```python
from build123d import *

# Parameters (mm, degrees)
ESQUISSE1_R             = 20
ESQUISSE1_R_2           = 17
ESQUISSE1_R_3           = 15
BOSS_EXTRU_1_DEPTH      = 7.5
ESQUISSE1_3_R           = 15
ESQUISSE1_3_R_2         = 4
BOSS_EXTRU_2_DEPTH      = 6.5
ESQUISSE1_6_R           = 4
ESQUISSE1_6_R_2         = 2.5
BOSS_EXTRU_3_DEPTH      = 6.3
CONG_1_R                = 2
ESQUISSE4_R             = 2
ENL_V_MAT_EXTRU_1_DEPTH = 1.5
ESQUISSE3_R             = 1
ENL_V_MAT_EXTRU_2_DEPTH = 7.5
CONG_1_OF_SYM_TRIE1_R   = 2


with BuildPart() as part:
    # Esquisse1 → Boss.-Extru.1 (new body)
    # profile 1 of 2: a face of its own
    with BuildSketch(Plane.XY):
        Circle(ESQUISSE1_R)
        Circle(ESQUISSE1_R_2, mode=Mode.SUBTRACT)
    # profile 2 of 2: a face of its own
    with BuildSketch(Plane.XY):
        Circle(ESQUISSE1_R_2)
        Circle(ESQUISSE1_R_3, mode=Mode.SUBTRACT)
    boss_extru_1 = extrude(amount=BOSS_EXTRU_1_DEPTH)

    # Esquisse1<3> → Boss.-Extru.2 (add)
    with BuildSketch(Plane.XY):
        Circle(ESQUISSE1_3_R)
        with Locations(Location((0, 0, 0), (0, 0, 180))):
            Circle(ESQUISSE1_3_R_2, mode=Mode.SUBTRACT)
    boss_extru_2 = extrude(amount=BOSS_EXTRU_2_DEPTH)

    # Esquisse1<6> → Boss.-Extru.3 (add)
    with BuildSketch(Plane.XY):
        with Locations(Location((0, 0, 0), (0, 0, 180))):
            Circle(ESQUISSE1_6_R)
        Circle(ESQUISSE1_6_R_2, mode=Mode.SUBTRACT)
    boss_extru_3 = extrude(amount=BOSS_EXTRU_3_DEPTH)

    # Congé1
    # the kernel refuses this fillet: 2 mm, written as the material it takes off along each edge
    with BuildSketch(Plane(origin=(0, 0, 7.5), x_dir=(1, 0, 0), z_dir=(0, -1, 0))) as cong_1_piece_1:
        with BuildLine():
            CenterArc((16.732050808, -2), CONG_1_R, 90, 60)
            Line((15, -1), (14.965358984, -0.98))
            ThreePointArc((14.965358984, -0.98), (14.96, -0.5), (14.96, 0))
            Line((14.96, 0), (15, 0.04))
            Line((15, 0.04), (16.732050808, 0.04))
            Line((16.732050808, 0.04), (16.732050808, 0))
        make_face()
    revolve(axis=Axis((0, 0, 7.5), (0, 0, 1)), mode=Mode.SUBTRACT)

    # Esquisse4 → Enlèv. mat.-Extru.1 (cut)
    with BuildSketch(Plane.XY.offset(6.5)):
        with Locations((-10, 0)):
            Circle(ESQUISSE4_R)
        with Locations((-5, 8.660254038)):
            Circle(ESQUISSE4_R)
        with Locations((5, 8.660254038)):
            Circle(ESQUISSE4_R)
        with Locations((10, 0)):
            Circle(ESQUISSE4_R)
        with Locations((5, -8.660254038)):
            Circle(ESQUISSE4_R)
        with Locations((-5, -8.660254038)):
            Circle(ESQUISSE4_R)
    enl_v_mat_extru_1 = extrude(amount=-ENL_V_MAT_EXTRU_1_DEPTH, mode=Mode.SUBTRACT)

    # Esquisse3 → Enlèv. mat.-Extru.2 (cut)
    with BuildSketch(Plane.XY.offset(6.5)):
        with Locations((0, 12.5)):
            Circle(ESQUISSE3_R)
        with Locations((-10.825317547, 6.25)):
            Circle(ESQUISSE3_R)
        with Locations((-10.825317547, -6.25)):
            Circle(ESQUISSE3_R)
        with Locations((0, -12.5)):
            Circle(ESQUISSE3_R)
        with Locations((10.825317547, -6.25)):
            Circle(ESQUISSE3_R)
        with Locations((10.825317547, 6.25)):
            Circle(ESQUISSE3_R)
    enl_v_mat_extru_2 = extrude(amount=-ENL_V_MAT_EXTRU_2_DEPTH, mode=Mode.SUBTRACT)

    # Symétrie1: Boss.-Extru.1, Boss.-Extru.2, Boss.-Extru.3, Enlèv. mat.-Extru.1, Enlèv. mat.-Extru.2 across plane
    add(boss_extru_1.mirror(Plane.XY))
    add(boss_extru_2.mirror(Plane.XY))
    add(boss_extru_3.mirror(Plane.XY))
    add(enl_v_mat_extru_1.mirror(Plane.XY), mode=Mode.SUBTRACT)
    add(enl_v_mat_extru_2.mirror(Plane.XY), mode=Mode.SUBTRACT)

    # Congé1 of Symétrie1
    # the kernel refuses this fillet: 2 mm, written as the material it takes off along each edge
    with BuildSketch(Plane(origin=(0, 0, -7.5), x_dir=(1, 0, 0), z_dir=(0, -1, 0))) as cong_1_of_sym_trie1_piece_1:
        with BuildLine():
            CenterArc((16.732050808, 2), CONG_1_OF_SYM_TRIE1_R, 210, 60)
            Line((15, 1), (14.965358984, 0.98))
            ThreePointArc((14.965358984, 0.98), (14.96, 0.5), (14.96, 0))
            Line((14.96, 0), (15, -0.04))
            Line((15, -0.04), (16.732050808, -0.04))
            Line((16.732050808, -0.04), (16.732050808, 0))
        make_face()
    revolve(axis=Axis((0, 0, -7.5), (0, 0, 1)), mode=Mode.SUBTRACT)


solid = part.part
```
Verification items for the finished model (mm, model axes). A direction names the side the tool comes from. Round coordinates to 2 decimals unless told otherwise and drop trailing zeros. Write each loop counter-clockwise with the first axis right and the second up, starting at its lowest first coordinate (ties: lowest second). Pieces come first, ordered by that corner, then holes. Notation, with made-up numbers: (-19, -8.75) -> (-4, -8.75) arc R15 cw to (-4, -0.75) -> close; hole circle Ø10 at (-6.5, 4.25). An arc over 180 degrees is marked (long way). Write each question's results on one line, items separated by ' | '. Start each with the question number.
1. Set-up check for faces 1 (the flat face through (-5, -9, 5)), 2 (the flat face through (-12, -12, -7.5)), 3 (the flat face through (-5, -9, -5)): record each of +Z, -Z, +X, -X, +Y, -Y from which the full face is reachable in a straight line by a thin tool's end or side.
2. Depth check by flat-ended pin: P1, Ø2.5, axis at x = 10, y = 0, coming from the +Z side; P2, Ø3, axis at y = 8.5, z = 3, coming from the +X side (3 decimals); P3, Ø6, axis at x = -9.5, y = -0.5, coming from the +Z side. Enter the tip coordinate at first touch or a pass-through.
3. Cross-section at A-A (z = -1). Enter the section's corners in (x, y).
4. Material ranges on probe 1 along Y at (x, z) = (0, -5); probe 2 along Z at (x, y) = (-1, 14); probe 3 along Y at (x, z) = (-10.5, -0.5), recorded low to high. Write a range as from..to.
5. Cross-section at B-B (x = 17.5). Enter the section's corners in (y, z), then the cut area to 3 significant figures.
6. Draft check along X on faces 4 (the cylindrical face through (3, -8.6, 5.8)), 5 (the cylindrical face through (-4.336, -19.524, 0.105)), 6 (the flat face through (-12, -12, 7.5)), 7 (the flat face through (10, 0, -5)). Enter one of: +X half, -X half, draft (parallel to the pull), parting line (faces both ways), or undercut.
Solutions:
1) face 1: +Z | face 2: -Z, +X, -X, +Y, -Y | face 3: -Z
2) P1: stops at z = 5 | P2: stops at x = 18.735 | P3: stops at z = 6.5
3) outline: circle Ø40 at (0, 0); hole circle Ø2 at (-10.83, -6.25); hole circle Ø2 at (-10.83, 6.25); hole circle Ø5 at (0, 0); hole circle Ø2 at (0, -12.5); hole circle Ø2 at (0, 12.5); hole circle Ø2 at (10.83, -6.25); hole circle Ø2 at (10.83, 6.25)
4) probe 1: y = -20..-13.5, -11.5..-2.5, 2.5..11.5, 13.5..20 | probe 2: z = -6.5..6.5 | probe 3: y = -17.02..-7.2, -5.3..5.3, 7.2..17.02
5) outline: (-9.68, -7.5) -> (9.68, -7.5) -> (9.68, 7.5) -> (-9.68, 7.5) -> close | area: 290 mm2
6) face 4: undercut | face 5: parting line | face 6: draft | face 7: undercut
